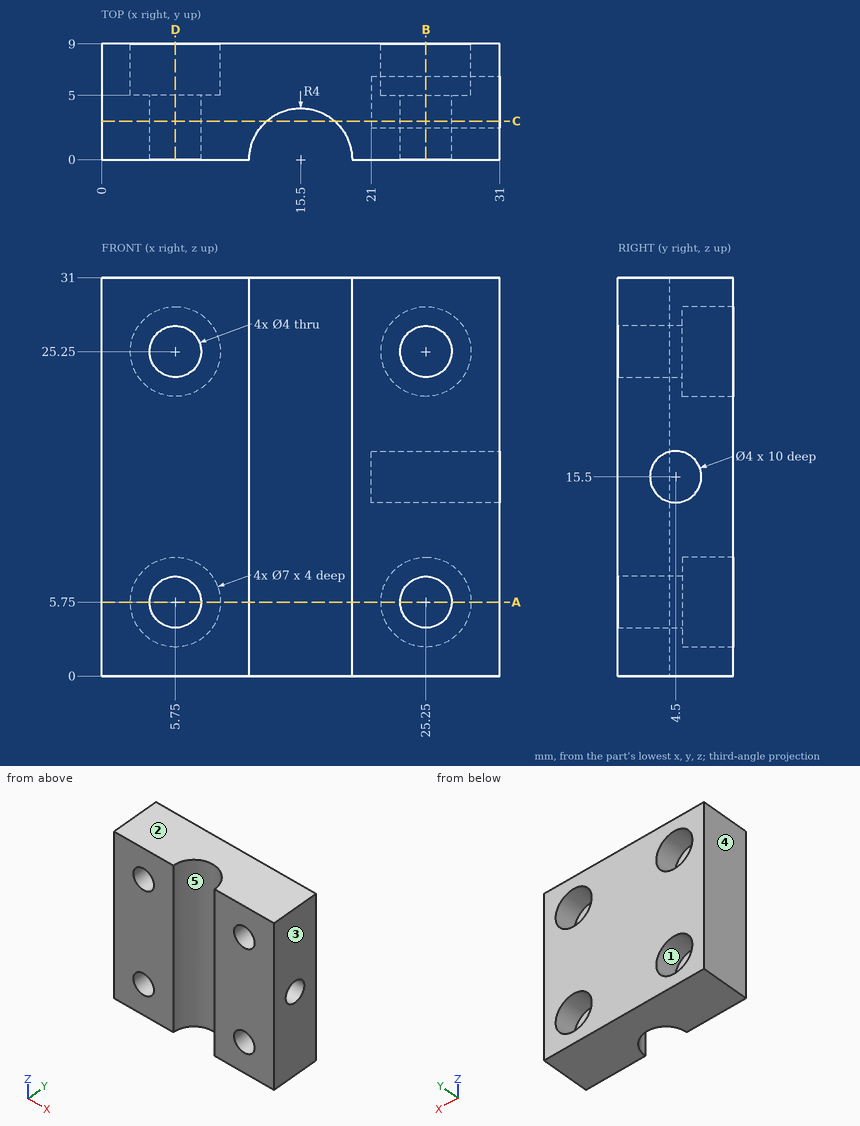
Drawing for the job (mm, zero at the part's lowest x, y, z). A direction names the side the tool comes from. Coordinates: 2 decimals unless noted, no trailing zeros. Order: outer loops, then holes, each group sorted by start corner. A loop starts at its lowest first (then second) coordinate and runs counter-clockwise, first axis right, second up. Notation, with made-up numbers: (-3, 15) - (53, 15) arc R4 cw to (53, 22) - close; hole circle Ø3 at (-17, 56). An arc over 180 degrees is marked (long way). Use a Markdown table: item, result. Add a question column.
(1) Saw through at B-B (x = 25.25). Give the cut face in (y, z).
(2) Which spindle directions (+Z, -Z, +X, -X, +Y, -Y) get a long thin tool onto all of the face, cutting with end or side? Do the marked faces 1 and 2. Say none if no direction does.
(3) Saw through at C-C (y = 3). Give the cut face in (x, z).
(4) Drill centre lines: line 1 along X through (y, z) = (6.3, 25.25); line 2 along X through (y, z) = (1.95, 25.25); line 3 along X through (y, z) = (4.5, 24). Where is each one in solid material? Low to high. Write a range as [from, to].
(5) Saw through at A-A (z = 5.75). Give the cut face in (x, y).
(6) Saw through at D-D (x = 5.75). Give the cut face in (y, z), then the cut area to 3 significant figures.
(7) Pull direction X, two halves, no side cores. Call the marked faces 3, 4 and 5: +X half, -X half, draft (parallel to the pull), parting line (faces both ways), or undercut.
(8) Flat gauge pins, fed straight in: pin 1 (3.5 mm diameter, centred on x = 7, z = 24.5, fed in from +Y); pin 2 (5.5 mm diameter, centred on x = 7, z = 5, fed in from +Y); pin 3 (3.5 mm diameter, centred on x = 5.75, z = 5.75, fed in from -Y). Where does each tip first touch, or does it go through?
Solved:
| question | item | result |
|---|---|---|
| 1 | outline | (0, 0) - (9, 0) - (9, 2.25) - (5, 2.25) - (5, 3.75) - (0, 3.75) - close; (0, 7.75) - (5, 7.75) - (5, 9.25) - (9, 9.25) - (9, 21.75) - (5, 21.75) - (5, 23.25) - (0, 23.25) - close; (0, 27.25) - (5, 27.25) - (5, 28.75) - (9, 28.75) - (9, 31) - (0, 31) - close; hole circle Ø4 at (4.5, 15.5) |
| 2 | face 1 | +Y |
| 2 | face 2 | +Z, +X, -X, +Y, -Y |
| 3 | outline | (0, 0) - (12.85, 0) - (12.85, 31) - (0, 31) - close; (18.15, 0) - (31, 0) - (31, 14.18) - (21, 14.18) - (21, 16.82) - (31, 16.82) - (31, 31) - (18.15, 31) - close; hole circle Ø4 at (5.75, 5.75); hole circle Ø4 at (5.75, 25.25); hole circle Ø4 at (25.25, 5.75); hole circle Ø4 at (25.25, 25.25) |
| 4 | line 1 | x = [0, 2.25], [9.25, 21.75], [28.75, 31] |
| 4 | line 2 | x = [0, 3.75], [7.75, 12.01], [18.99, 23.25], [27.25, 31] |
| 4 | line 3 | x = [0, 4.19], [7.31, 23.69], [26.81, 31] |
| 5 | outline | (0, 0) - (3.75, 0) - (3.75, 5) - (2.25, 5) - (2.25, 9) - (0, 9) - close; (7.75, 0) - (11.5, 0) arc R4 cw to (19.5, 0) - (23.25, 0) - (23.25, 5) - (21.75, 5) - (21.75, 9) - (9.25, 9) - (9.25, 5) - (7.75, 5) - close; (27.25, 0) - (31, 0) - (31, 9) - (28.75, 9) - (28.75, 5) - (27.25, 5) - close |
| 6 | outline | (0, 0) - (9, 0) - (9, 2.25) - (5, 2.25) - (5, 3.75) - (0, 3.75) - close; (0, 7.75) - (5, 7.75) - (5, 9.25) - (9, 9.25) - (9, 21.75) - (5, 21.75) - (5, 23.25) - (0, 23.25) - close; (0, 27.25) - (5, 27.25) - (5, 28.75) - (9, 28.75) - (9, 31) - (0, 31) - close |
| 6 | area | 183 mm² |
| 7 | face 3 | +X half |
| 7 | face 4 | -X half |
| 7 | face 5 | undercut |
| 8 | pin 1 | stops at y = 5 |
| 8 | pin 2 | stops at y = 9 |
| 8 | pin 3 | passes through |
